```python
from build123d import *


with BuildPart() as part:
    # 草图1 → 旋转1 (revolve)
    with BuildSketch(Plane.XY, mode=Mode.PRIVATE) as revolve_1_sk:
        Polygon((0, 0), (0, 4), (15, 4), (15, 5), (16, 5), (16, 4.5), (17, 4.5), (17, 5), (22, 5), (22, 6), (29, 6), (29, 7), (30, 7), (30, 6.5), (31, 6.5), (31, 7), (51, 7), (51, 9), (53, 9), (53, 6), (64, 6), (64, 5), (69, 5), (69, 4.5), (70, 4.5), (70, 5), (71, 5), (71, 0), align=None)
    revolve(revolve_1_sk.sketch.rotate(Axis((0, 0, 0), (1, 0, 0)), 90), axis=Axis((0, 0, 0), (1, 0, 0)))


solid = part.part
```
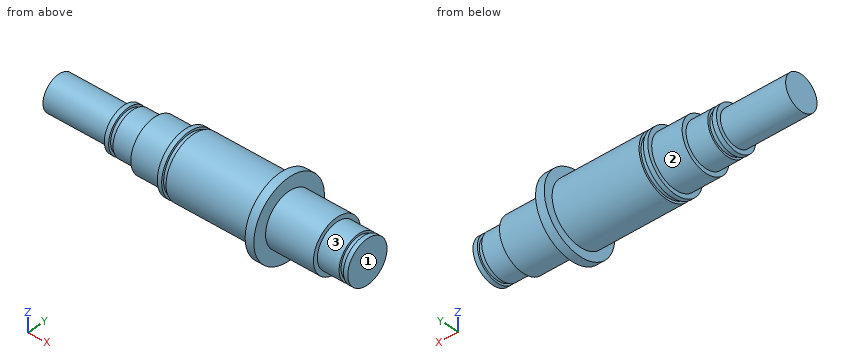
Design review of the part built by this model. Coordinates are the model's own, in mm. Face numbers are marked on the shaded views. A direction names the side the tool comes from. Give positions to 0.01 mm unless a question says otherwise; leave off trailing zeros. Order: outer loops, then holes, each group sorted by start corner. A loop starts at its lowest first (then second) coordinate and runs counter-clockwise, first axis right, second up. Notation, with made-up numbers: M 72.5,-16.75 L 129.5,-16.75 A20 ccw 129.5,9.25 Z; hole C 87.5,-27 d7. An arc over 180 degrees is marked long. One line per question, with ' | ' between items. Start each with the question number.
Q1. We need section A-A (x = 34). Write out the cut boundary in (y, z), plus the area to 3 significant figures.
Q2. For L1, parallel to X at y = 1.5, z = -4.5; L2, parallel to X at y = -8, z = -2.75; L3, parallel to X at y = -3, z = 2.75, list the stretches that pass through material, from the lowest coordinate up. Write a range as [from, to].
Q3. We need section B-B (x = 66). Write out the cut boundary in (y, z), plus the area to 3 significant figures.
Q4. For pin 1 Ø10 at (x, z) = (44.5, -4) entering from +Y; pin 2 Ø8 at (y, z) = (6, -7) entering from +X; pin 3 Ø2 at (x, y) = (43, -4.5) entering from -Z, all flat-tipped, find the tip position at first contact; note any pin that passes through.
Q5. Machinability: for the marked faces 1, 2 and 3, which of the approach directions +Z, -Z, +X, -X, +Y, -Y give a long, thin tool a straight path to every point of the face, cutting with its end or side? Answer none if there is none.
Returned:
1) outline: C 0,0 d14 | area: 154 mm2
2) L1: [15, 16], [17, 69], [70, 71] | L2: [51, 53] | L3: [15, 71]
3) outline: C 0,0 d10 | area: 78.5 mm2
4) pin 1: y = 7 | pin 2: x = 64 | pin 3: z = -6.06
5) face 1: +Z, -Z, +X, +Y, -Y | face 2: -X | face 3: +X
